The model under review builds one solid part; all positions refer to its coordinate system, in mm. Face numbers are marked on the shaded views. A direction names the side the tool comes from. Give positions to 0.01 mm unless a question says otherwise; leave off trailing zeros. Order: outer loops, then holes, each group sorted by start corner. A loop starts at its lowest first (then second) coordinate and runs counter-clockwise, first axis right, second up.
```python
from build123d import *

# Parameters (mm, degrees)
F1_DEPTH     = 5
F2_C1_SIZE2  = 0.25
F2_C1_SIZE   = 0.5
F2_C2_SIZE2  = 0.5
F2_C2_SIZE   = 0.25
F2_C3_SIZE2  = 0.5
F2_C3_SIZE   = 0.25
F2_C4_SIZE2  = 0.5
F2_C4_SIZE   = 0.25
F2_C5_SIZE2  = 0.25
F2_C5_SIZE   = 0.5
F2_C6_SIZE2  = 0.5
F2_C6_SIZE   = 0.25
F2_C7_SIZE2  = 0.5
F2_C7_SIZE   = 0.25
F2_C8_SIZE2  = 0.5
F2_C8_SIZE   = 0.25
F2_C9_SIZE2  = 0.5
F2_C9_SIZE   = 0.25
F2_C10_SIZE2 = 0.5
F2_C10_SIZE  = 0.25


with BuildPart() as f1:
    # F0 (on Top) → F1 (new body)
    with BuildSketch(Plane.XY):
        with BuildLine():
            Line((1.236000562, -12.0934582279), (0.4769388315, -14.1789632613))
            ThreePointArc((0.4769388315, -14.1789632613), (0.3854097856, -14.2982462382), (0.2420156754, -14.3434582279))
            Line((0.2420156754, -14.3434582279), (0.065349562, -14.3434582279))
            Line((0.065349562, -14.3434582279), (0.065349562, -17.3434582279))
            Line((0.065349562, -17.3434582279), (15.773299562, -17.3434582279))
            Line((15.773299562, -17.3434582279), (15.773299562, -14.3434582279))
            Line((15.773299562, -14.3434582279), (15.5966334485, -14.3434582279))
            ThreePointArc((15.5966334485, -14.3434582279), (15.4532393383, -14.2982462382), (15.3617102924, -14.1789632613))
            Line((15.3617102924, -14.1789632613), (14.602648562, -12.0934582279))
            Line((14.602648562, -12.0934582279), (13.802360562, -12.0934582279))
            Line((13.802360562, -12.0934582279), (13.0432988315, -14.1789632613))
            ThreePointArc((13.0432988315, -14.1789632613), (12.9517697856, -14.2982462382), (12.8083756754, -14.3434582279))
            Line((12.8083756754, -14.3434582279), (12.4550434485, -14.3434582279))
            ThreePointArc((12.4550434485, -14.3434582279), (12.3116493383, -14.2982462382), (12.2201202924, -14.1789632613))
            Line((12.2201202924, -14.1789632613), (11.461058562, -12.0934582279))
            Line((11.461058562, -12.0934582279), (10.660770562, -12.0934582279))
            Line((10.660770562, -12.0934582279), (9.9017088315, -14.1789632613))
            ThreePointArc((9.9017088315, -14.1789632613), (9.8101797856, -14.2982462382), (9.6667856754, -14.3434582279))
            Line((9.6667856754, -14.3434582279), (9.3134534485, -14.3434582279))
            ThreePointArc((9.3134534485, -14.3434582279), (9.1700593383, -14.2982462382), (9.0785302924, -14.1789632613))
            Line((9.0785302924, -14.1789632613), (8.319468562, -12.0934582279))
            Line((8.319468562, -12.0934582279), (7.519180562, -12.0934582279))
            Line((7.519180562, -12.0934582279), (6.7601188315, -14.1789632613))
            ThreePointArc((6.7601188315, -14.1789632613), (6.6685897856, -14.2982462382), (6.5251956754, -14.3434582279))
            Line((6.5251956754, -14.3434582279), (6.1718634485, -14.3434582279))
            ThreePointArc((6.1718634485, -14.3434582279), (6.0284693383, -14.2982462382), (5.9369402924, -14.1789632613))
            Line((5.9369402924, -14.1789632613), (5.177878562, -12.0934582279))
            Line((5.177878562, -12.0934582279), (4.377590562, -12.0934582279))
            Line((4.377590562, -12.0934582279), (3.6185288315, -14.1789632613))
            ThreePointArc((3.6185288315, -14.1789632613), (3.5269997856, -14.2982462382), (3.3836056754, -14.3434582279))
            Line((3.3836056754, -14.3434582279), (3.0302734485, -14.3434582279))
            ThreePointArc((3.0302734485, -14.3434582279), (2.8868793383, -14.2982462382), (2.7953502924, -14.1789632613))
            Line((2.7953502924, -14.1789632613), (2.036288562, -12.0934582279))
            Line((2.036288562, -12.0934582279), (1.236000562, -12.0934582279))
        make_face()
    extrude(amount=F1_DEPTH)

    # F2: chamfer of 0.25 x 0.5 on 10 edges, made by hand

    # F2_c1
    f2_c1_edges = [f1.edges().sort_by_distance(p)[0] for p in [
        (7.919324562, -12.0934582279, 0),
    ]]
    f2_c1_side = f1.faces().sort_by_distance((7.919324562, -12.0934582279, 0.005))[0]
    chamfer(f2_c1_edges, length=F2_C1_SIZE, length2=F2_C1_SIZE2, reference=f2_c1_side)

    # F2_c2
    f2_c2_edges = [f1.edges().sort_by_distance(p)[0] for p in [
        (7.919324562, -12.0934582279, 5),
    ]]
    f2_c2_side = f1.faces().sort_by_distance((7.919324562, -12.0934582279, 4.995))[0]
    chamfer(f2_c2_edges, length=F2_C2_SIZE, length2=F2_C2_SIZE2, reference=f2_c2_side)

    # F2_c3
    f2_c3_edges = [f1.edges().sort_by_distance(p)[0] for p in [
        (4.777734562, -12.0934582279, 0),
    ]]
    f2_c3_side = f1.faces().sort_by_distance((4.777734562, -12.0984582279, 0))[0]
    chamfer(f2_c3_edges, length=F2_C3_SIZE, length2=F2_C3_SIZE2, reference=f2_c3_side)

    # F2_c4
    f2_c4_edges = [f1.edges().sort_by_distance(p)[0] for p in [
        (4.777734562, -12.0934582279, 5),
    ]]
    f2_c4_side = f1.faces().sort_by_distance((4.777734562, -12.0934582279, 4.995))[0]
    chamfer(f2_c4_edges, length=F2_C4_SIZE, length2=F2_C4_SIZE2, reference=f2_c4_side)

    # F2_c5
    f2_c5_edges = [f1.edges().sort_by_distance(p)[0] for p in [
        (1.636144562, -12.0934582279, 0),
    ]]
    f2_c5_side = f1.faces().sort_by_distance((1.636144562, -12.0984582279, 0))[0]
    chamfer(f2_c5_edges, length=F2_C5_SIZE, length2=F2_C5_SIZE2, reference=f2_c5_side)

    # F2_c6
    f2_c6_edges = [f1.edges().sort_by_distance(p)[0] for p in [
        (1.636144562, -12.0934582279, 5),
    ]]
    f2_c6_side = f1.faces().sort_by_distance((1.636144562, -12.0934582279, 4.995))[0]
    chamfer(f2_c6_edges, length=F2_C6_SIZE, length2=F2_C6_SIZE2, reference=f2_c6_side)

    # F2_c7
    f2_c7_edges = [f1.edges().sort_by_distance(p)[0] for p in [
        (14.202504562, -12.0934582279, 0),
    ]]
    f2_c7_side = f1.faces().sort_by_distance((14.202504562, -12.0984582279, 0))[0]
    chamfer(f2_c7_edges, length=F2_C7_SIZE, length2=F2_C7_SIZE2, reference=f2_c7_side)

    # F2_c8
    f2_c8_edges = [f1.edges().sort_by_distance(p)[0] for p in [
        (14.202504562, -12.0934582279, 5),
    ]]
    f2_c8_side = f1.faces().sort_by_distance((14.202504562, -12.0934582279, 4.995))[0]
    chamfer(f2_c8_edges, length=F2_C8_SIZE, length2=F2_C8_SIZE2, reference=f2_c8_side)

    # F2_c9
    f2_c9_edges = [f1.edges().sort_by_distance(p)[0] for p in [
        (11.060914562, -12.0934582279, 0),
    ]]
    f2_c9_side = f1.faces().sort_by_distance((11.060914562, -12.0984582279, 0))[0]
    chamfer(f2_c9_edges, length=F2_C9_SIZE, length2=F2_C9_SIZE2, reference=f2_c9_side)

    # F2_c10
    f2_c10_edges = [f1.edges().sort_by_distance(p)[0] for p in [
        (11.060914562, -12.0934582279, 5),
    ]]
    f2_c10_side = f1.faces().sort_by_distance((11.060914562, -12.0934582279, 4.995))[0]
    chamfer(f2_c10_edges, length=F2_C10_SIZE, length2=F2_C10_SIZE2, reference=f2_c10_side)


solid = f1.part
```
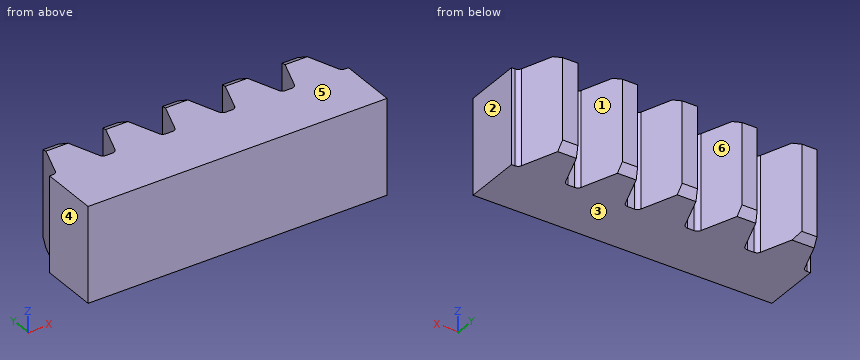
1. Take a section at B-B (y = -13.6). Write out the cut boundary in (x, z).
2. Draft analysis for pull direction X (two halves, no side actions). For the marked faces 1, 2, 3 and 4, state which applies: pulls with the +X half, pulls with the -X half, needs draft (parallel to the pull), parting line crosses it, or undercut.
3. Take a section at C-C (x = 9.5). Write out the cut boundary in (y, z).
4. To check wall thickness, follow line 1 (X direction, y = -14.2, z = 1.45); line 2 (X direction, y = -13.45, z = 3.05); line 3 (Y direction, x = 12.5, z = 2.1). State the ranges of each line that lie inside material, in increasing order.
5. For the marked faces 5 and 6, list the 3-axis set-ups (+Z, -Z, +X, -X, +Y, -Y) from which the entire face can be reached by the end or side of a thin tool; tool diameter is ignored.
Answer:
1. outline: (0.69, 0) - (2.58, 0) - (2.58, 5) - (0.69, 5) - close; (3.83, 0) - (5.73, 0) - (5.73, 5) - (3.83, 5) - close; (6.97, 0) - (8.87, 0) - (8.87, 5) - (6.97, 5) - close; (10.11, 0) - (12.01, 0) - (12.01, 5) - (10.11, 5) - close; (13.25, 0) - (15.15, 0) - (15.15, 5) - (13.25, 5) - close
2. face 1: undercut
2. face 2: pulls with the +X half
2. face 3: needs draft
2. face 4: pulls with the -X half
3. outline: (-17.34, 0) - (-14.34, 0) - (-14.34, 5) - (-17.34, 5) - close
4. line 1: x = 0.47 to 2.8, 3.61 to 5.95, 6.75 to 9.09, 9.89 to 12.23, 13.03 to 15.37
4. line 2: x = 0.74 to 2.53, 3.88 to 5.67, 7.03 to 8.81, 10.17 to 11.95, 13.31 to 15.1
4. line 3: y = -17.34 to -14.34
5. face 5: +Z, +X, -X, +Y, -Y
5. face 6: +Z, -Z, +Y
